Check sheet for the modelled part. Datum: model origin and axes. Units: mm. A direction names the side the tool comes from. Round coordinates to 2 decimals unless told otherwise and drop trailing zeros. Write each loop counter-clockwise with the first axis right and the second up, starting at its lowest first coordinate (ties: lowest second). Pieces come first, ordered by that corner, then holes. Notation, with made-up numbers: (86, 62.25) -> (104, 62.25) arc R23 cw to (104, 78.25) -> close; hole circle Ø10 at (-11, -39). An arc over 180 degrees is marked (long way). One line per item, written item: value. Start each with the question number.
```python
from build123d import *

# Parameters (mm, degrees)
SKETCH1_R           = 28.575
BOSS_EXTRUDE1_DEPTH = 397
SKETCH2_R           = 24.5
BOSS_EXTRUDE2_DEPTH = 55
SKETCH3_R           = 20.64
BOSS_EXTRUDE3_DEPTH = 40
SKETCH4_R           = 18.9
BOSS_EXTRUDE4_DEPTH = 38
FILLET1_R           = 1
SKETCH5_R           = 5
BOSS_EXTRUDE5_DEPTH = 5


with BuildPart() as part:
    # Sketch1 → Boss-Extrude1 (new body)
    with BuildSketch(Plane(origin=(0, 0, 0), x_dir=(1, 0, 0), z_dir=(0, 1, 0))):
        with Locations(Location((0, 0, 0), (0, 0, 270))):
            Circle(SKETCH1_R)
    extrude(amount=BOSS_EXTRUDE1_DEPTH)

    # Sketch2 → Boss-Extrude2 (add)
    with BuildSketch(Plane(origin=(0, 397, 0), x_dir=(1, 0, 0), z_dir=(0, 1, 0))):
        with Locations(Location((0, 0, 0), (0, 0, 270))):
            Circle(SKETCH2_R)
    extrude(amount=BOSS_EXTRUDE2_DEPTH)

    # Sketch3 → Boss-Extrude3 (add)
    with BuildSketch(Plane(origin=(0, 452, 0), x_dir=(1, 0, 0), z_dir=(0, 1, 0))):
        with Locations(Location((0, 0, 0), (0, 0, 270))):
            Circle(SKETCH3_R)
    extrude(amount=BOSS_EXTRUDE3_DEPTH)

    # Sketch4 → Boss-Extrude4 (add)
    with BuildSketch(Plane(origin=(0, 492, 0), x_dir=(1, 0, 0), z_dir=(0, 1, 0))):
        with Locations(Location((0, 0, 0), (0, 0, 270))):
            Circle(SKETCH4_R)
    extrude(amount=BOSS_EXTRUDE4_DEPTH)

    # Fillet1
    fillet1_edges = [part.edges().sort_by_distance(p)[0] for p in [
        (0, 492, -20.64),
        (0, 530, -18.9),
        (0, 397, -28.575),
        (0, 452, -24.5),
    ]]
    fillet(fillet1_edges, radius=FILLET1_R)

    # Sketch5 → Boss-Extrude5 (add)
    with BuildSketch(Plane.XZ):
        with Locations(Location((0, 0, 0), (0, 0, 270))):
            Circle(SKETCH5_R)
    extrude(amount=BOSS_EXTRUDE5_DEPTH)


solid = part.part
```
1. Cross-section at D-D (y = 437). Record the cut outline in (x, z).
2. Access from +Z, -Z, +X, -X, +Y, -Y to the whole of each face (thin tool, end or side, straight path). Record for faces 1 (the face through (10.3, 492, -16.1)), 2 (the face through (-4.88, -2.46, 1.08)), 3 (the face through (0, 530, 0)).
3. Depth check by flat-ended pin: pin 1 Ø1.5 at (x, y) = (-14.5, 322.5) entering from -Z; pin 2 Ø2 at (x, y) = (-8, 473) entering from +Z; pin 3 Ø6 at (x, y) = (5, 257) entering from +Z. Enter the tip coordinate at first touch or a pass-through.
4. Material ranges on probe 1 along Y at (x, z) = (-6, 4); probe 2 along X at (y, z) = (467, -6.5); probe 3 along Y at (x, z) = (7, 22.5), recorded low to high.
5. Cross-section at C-C (y = 233.5). Record the cut outline in (x, z) (3 decimals), plus the area to 3 significant figures.
6. Cross-section at B-B (z = 0). Record the cut outline in (x, y) (3 decimals).
7. Cross-section at A-A (x = 0). Record the cut outline in (y, z) (3 decimals).
Working result:
1. outline: circle Ø49 at (0, 0)
2. face 1: +Y
2. face 2: -Y
2. face 3: +Z, -Z, +X, -X, +Y
3. pin 1: stops at z = -25.05
3. pin 2: stops at z = 19.42
3. pin 3: stops at z = 28.5
4. probe 1: y = 0 to 530
4. probe 2: x = -19.59 to 19.59
4. probe 3: y = 0 to 452
5. outline: circle Ø57.15 at (0, 0)
5. area: 2,570 mm^2
6. outline: (-28.575, 0) -> (-5, 0) -> (-5, -5) -> (5, -5) -> (5, 0) -> (28.575, 0) -> (28.575, 396) arc R1 ccw to (27.575, 397) -> (24.5, 397) -> (24.5, 451) arc R1 ccw to (23.5, 452) -> (20.64, 452) -> (20.64, 491) arc R1 ccw to (19.64, 492) -> (18.9, 492) -> (18.9, 529) arc R1 ccw to (17.9, 530) -> (-17.9, 530) arc R1 ccw to (-18.9, 529) -> (-18.9, 492) -> (-19.64, 492) arc R1 ccw to (-20.64, 491) -> (-20.64, 452) -> (-23.5, 452) arc R1 ccw to (-24.5, 451) -> (-24.5, 397) -> (-27.575, 397) arc R1 ccw to (-28.575, 396) -> close
7. outline: (-5, -5) -> (0, -5) -> (0, -28.575) -> (396, -28.575) arc R1 ccw to (397, -27.575) -> (397, -24.5) -> (451, -24.5) arc R1 ccw to (452, -23.5) -> (452, -20.64) -> (491, -20.64) arc R1 ccw to (492, -19.64) -> (492, -18.9) -> (529, -18.9) arc R1 ccw to (530, -17.9) -> (530, 17.9) arc R1 ccw to (529, 18.9) -> (492, 18.9) -> (492, 19.64) arc R1 ccw to (491, 20.64) -> (452, 20.64) -> (452, 23.5) arc R1 ccw to (451, 24.5) -> (397, 24.5) -> (397, 27.575) arc R1 ccw to (396, 28.575) -> (0, 28.575) -> (0, 5) -> (-5, 5) -> close
